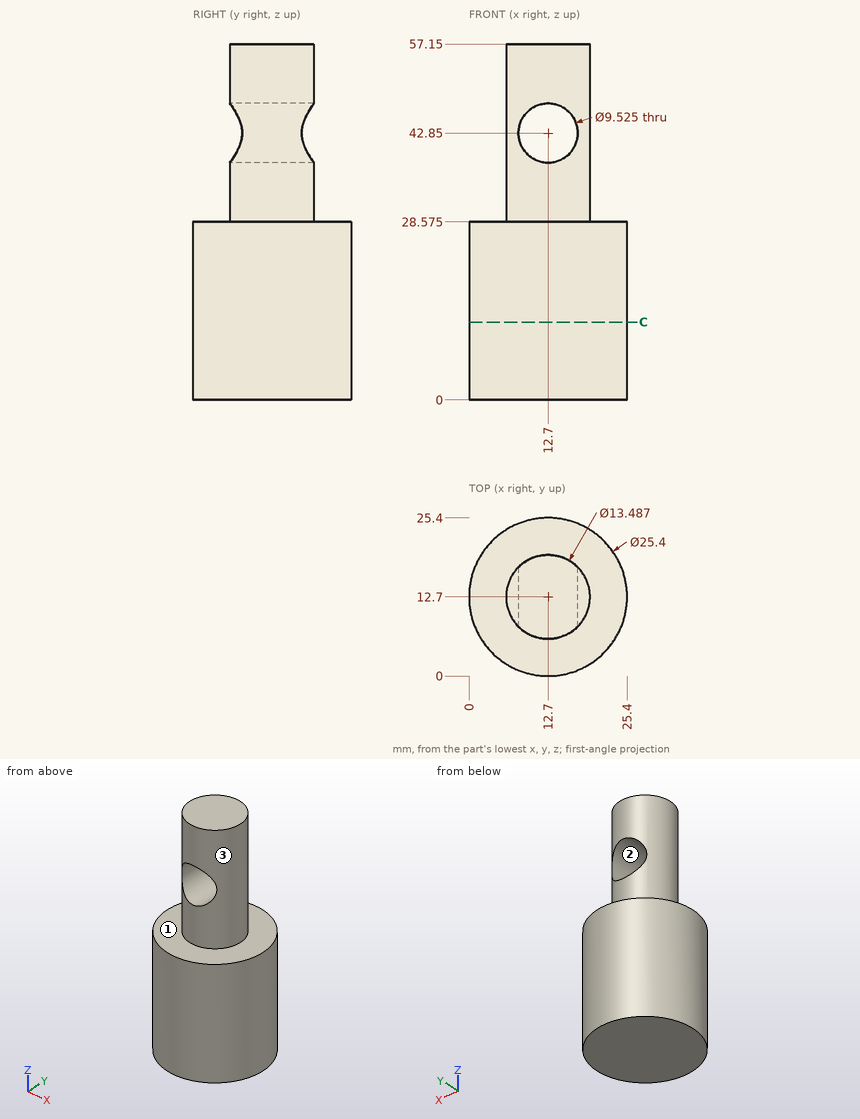
Geometry: see drawing. Coordinates: mm, zero at the bounding-box minimum. Give positions to 0.01 mm unless a question says otherwise; leave off trailing zeros. Order: outer loops, then holes, each group sorted by start corner. A loop starts at its lowest first (then second) coordinate and runs counter-clockwise, first axis right, second up.
1. Line query: probe 1 along Z at (x, y) = (12.7, 8.5); probe 2 along X at (y, z) = (12.5, 5.5); probe 3 along Z at (x, y) = (8, 3.5) (1 decimal). Output: solid intervals per line, ascending.
Computed:
probe 1: z = 0 to 38.09, 47.61 to 57.15
probe 2: x = 0 to 25.4
probe 3: z = 0 to 28.6
2. Draft query along X for the marked faces 1, 2 and 3. Return one class per face: released by +X, released by -X, zero draft, split by the parting line, or undercut.
Computed:
face 1: zero draft
face 2: undercut
face 3: split by the parting line
3. Pin query (flat end, axial travel): pin 1 Ø4 at (x, z) = (5, 33) entering from -Y (1 decimal); pin 2 Ø3 at (x, z) = (16.5, 17.5) entering from +Y; pin 3 Ø10 at (y, z) = (8, 42) entering from +X. Return the tip coordinate at first contact, or that it passes through.
Computed:
pin 1: stops at y = 9.1
pin 2: stops at y = 25.19
pin 3: stops at x = 19.44
4. Cut plane C-C (z = 12.5). Return loops of the section in (x, y), and give its area (3 significant figures).
Computed:
outline: circle Ø25.4 at (12.7, 12.7)
area: 507 mm2
